Design review of the part built by this model. Coordinates are the model's own, in mm. Face numbers are marked on the shaded views. A direction names the side the tool comes from. Coordinates: 2 decimals unless noted, no trailing zeros. Loops run counter-clockwise (first coordinate to the right, second up) from the corner with the lowest first, then second, coordinate; pieces in that order, holes last. Notation, with made-up numbers: M 44,39.25 L 83,39.25 A25 ccw 83,62.25 Z; hole C 25.25,-19 d3. An arc over 180 degrees is marked long. Answer as a JSON object with one key per item and string values. Group by question number.
1. Draft analysis for pull direction Y (two halves, no side actions). For the marked faces 1, 2 and 3, state which applies: +Y half, -Y half, draft (parallel to the pull), parting line (faces both ways), or undercut.
2. Consider section C-C (z = -3). State the section outline as (x, y) points.
3. Consider section D-D (z = 8.5). State the section outline as (x, y) points, then the cut area to 3 significant figures.
4. Consider section B-B (z = -8). State the section outline as (x, y) points, then the cut area to 3 significant figures.
5. Insertion check: pin 1 (3.5 mm diameter, centred on y = 0, z = -8, fed in from -X); pin 2 (5 mm diameter, centred on y = 20, z = 2, fed in from -X); pin 3 (3 mm diameter, centred on y = -20, z = -3, fed in from -X); pin 4 (10 mm diameter, centred on y = 1, z = -3, fed in from -X). Each pin has a flat end and moves straight along its axis. Give the tip position at first contact, or say it passes through.
6. Machinability: for the marked faces 4 and 5, which of the approach directions +Z, -Z, +X, -X, +Y, -Y give a long, thin tool a straight path to every point of the face, cutting with its end or side? Answer none if there is none.
7. Consider section A-A (x = 0). Count the separate pieces of the cut face and the enclosed holes in it, then the cut area to 3 significant figures.
8. To check wall thickness, follow probe 1 along Z at (x, y) = (-25, 0); probe 2 along Z at (x, y) = (15, -2.5); probe 3 along Z at (x, y) = (-1, 26). State the ranges of each line that lie inside material, in increasing order.
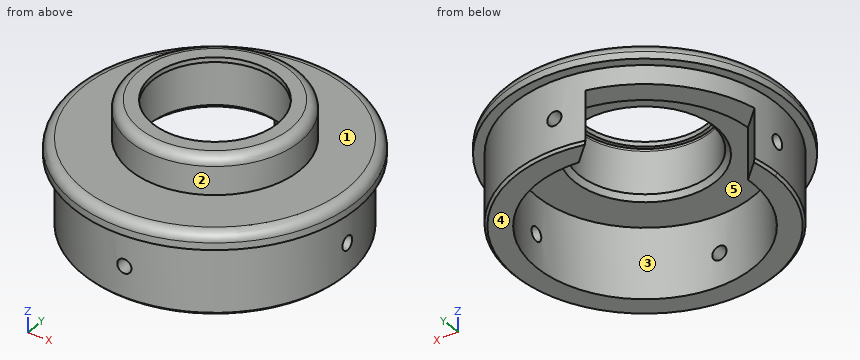
from build123d import *

# Parameters (mm, degrees)
SKETCH_2_R               = 30
SKETCH_2_R_2             = 14
EXTRUDE_1_DEPTH          = 11.5
EXTRUDE_START            = -1.5
SKETCH_3_R               = 14
SKETCH_3_R_2             = 13.25
EXTRUDE_2_DEPTH          = 1.5
SKETCH_4_R               = 33.760613234
SKETCH_4_R_2             = 18
CUT_EXTRUDE_1_DEPTH      = 8
FILLET_1_R               = 2
FILLET_2_R               = 2
SKETCH_6_R               = 28
SKETCH_6_R_2             = 23
EXTRUDE_3_DEPTH          = 15
CUT_EXTRUDE_2_DEPTH      = 46
CUT_EXTRUDE_2_DEPTH_BACK = 46
SKETCH_7_R               = 1.5
CUT_EXTRUDE_3_DEPTH      = 46.000000033
CUT_EXTRUDE_3_DEPTH_BACK = 46.000000033
SKETCH_8_R               = 1.5
CUT_EXTRUDE_4_DEPTH      = 11
SKETCH_15_R              = 14
CUT_EXTRUDE_5_DEPTH      = 0.5
CHAMFER_1_SIZE           = 1
CHAMFER_2_SIZE           = 0.5


with BuildPart() as part:
    # 스케치2 → 보스-돌출1 (new body)
    with BuildSketch(Plane.XY):
        Circle(SKETCH_2_R)
        Circle(SKETCH_2_R_2, mode=Mode.SUBTRACT)
    extrude(amount=EXTRUDE_1_DEPTH)

    # 스케치3 → 보스-돌출2 (add)
    with BuildSketch(Plane.XY.offset(11.5).offset(EXTRUDE_START)):
        Circle(SKETCH_3_R)
        Circle(SKETCH_3_R_2, mode=Mode.SUBTRACT)
    extrude(amount=EXTRUDE_2_DEPTH)

    # 스케치4 → 컷-돌출1 (cut)
    with BuildSketch(Plane.XY.offset(11.5)):
        Circle(SKETCH_4_R)
        Circle(SKETCH_4_R_2, mode=Mode.SUBTRACT)
    extrude(amount=-CUT_EXTRUDE_1_DEPTH, mode=Mode.SUBTRACT)

    # 필렛1
    fillet_1_edges = [part.edges().sort_by_distance(p)[0] for p in [
        (-18, 0, 11.5),
    ]]
    fillet(fillet_1_edges, radius=FILLET_1_R)

    # 필렛2
    fillet_2_edges = [part.edges().sort_by_distance(p)[0] for p in [
        (-30, 0, 3.5),
    ]]
    fillet(fillet_2_edges, radius=FILLET_2_R)

    # 스케치6 → 보스-돌출3 (add)
    with BuildSketch(Plane(origin=(0, 0, 0), x_dir=(-1, 0, 0), z_dir=(0, 0, -1))):
        Circle(SKETCH_6_R)
        Circle(SKETCH_6_R_2, mode=Mode.SUBTRACT)
    extrude(amount=EXTRUDE_3_DEPTH)

    # 스케치7 → 컷-돌출2 (cut, two sides: drawn at the far end of the back side and taken through both)
    with BuildSketch(Plane(origin=(0, 0, 0), x_dir=(1, 0, 0), z_dir=(0, 1, 0)).offset(-CUT_EXTRUDE_2_DEPTH_BACK)):
        with Locations(Location((0, 8, 0), (0, 0, 270))):
            Circle(SKETCH_7_R)
    extrude(amount=CUT_EXTRUDE_2_DEPTH + CUT_EXTRUDE_2_DEPTH_BACK, mode=Mode.SUBTRACT)

    # 스케치8 → 컷-돌출3 (cut, two sides: drawn at the far end of the back side and taken through both)
    with BuildSketch(Plane(origin=(0, 0, 0), x_dir=(0, 0, -1), z_dir=(1, 0, 0)).offset(-CUT_EXTRUDE_3_DEPTH_BACK)):
        with Locations((8, 0)):
            Circle(SKETCH_8_R)
    extrude(amount=CUT_EXTRUDE_3_DEPTH + CUT_EXTRUDE_3_DEPTH_BACK, mode=Mode.SUBTRACT)

    # 스케치13 → 컷-돌출4 (cut)
    with BuildSketch(Plane(origin=(0, 0, -15), x_dir=(-1, 0, 0), z_dir=(0, 0, -1))):
        Polygon((19.798989873, 19.798989873), (30.405591591, 9.192388155), (19.798989873, -1.414213562), (9.192388155, 9.192388155), (-1.414213562, 19.798989873), (9.192388155, 30.405591591), align=None)
    extrude(amount=-CUT_EXTRUDE_4_DEPTH, mode=Mode.SUBTRACT)

    # 스케치15 → 컷-돌출5 (cut)
    with BuildSketch(Plane(origin=(0, 0, 10), x_dir=(-1, 0, 0), z_dir=(0, 0, -1))):
        Circle(SKETCH_15_R)
    extrude(amount=-CUT_EXTRUDE_5_DEPTH, mode=Mode.SUBTRACT)

    # 모따기1
    chamfer_1_edges = [part.edges().sort_by_distance(p)[0] for p in [
        (-14, 0, 0),
    ]]
    chamfer(chamfer_1_edges, length=CHAMFER_1_SIZE)

    # 모따기2
    chamfer_2_edges = [part.edges().sort_by_distance(p)[0] for p in [
        (21.853217724, -17.505338474, -15),
    ]]
    chamfer(chamfer_2_edges, length=CHAMFER_2_SIZE)


solid = part.part
Findings below:
{
 "1": {"face 1": "draft", "face 2": "parting line", "face 3": "undercut"},
 "2": {"outline": "C 0,0 d56; hole C 0,0 d46"},
 "3": {"outline": "C 0,0 d36; hole C 0,0 d28", "area": "402 mm^2"},
 "4": {"outline": "M -27.96,-1.5 A28 ccw -1.5,-27.96 L -1.5,-22.95 A23 cw -22.95,-1.5 Z; M -27.96,1.5 L -22.95,1.5 A23 cw -22.94,1.72 L -27.32,6.11 A28 ccw Z; M -6.11,27.32 L -1.72,22.94 A23 cw -1.5,22.95 L -1.5,27.96 A28 ccw Z; M 1.5,-27.96 A28 ccw 27.96,-1.5 L 22.95,-1.5 A23 cw 1.5,-22.95 Z; M 1.5,22.95 A23 cw 22.95,1.5 L 27.96,1.5 A28 ccw 1.5,27.96 Z", "area": "581 mm^2"},
 "5": {"pin 1": "stops at x = -28", "pin 2": "stops at x = -24.34", "pin 3": "stops at x = -21.02", "pin 4": "stops at x = -30"},
 "6": {"face 4": "-Z, +X, -X, +Y, -Y", "face 5": "-Z"},
 "7": {"separate pieces": "4", "enclosed holes": "0", "area": "293 mm^2"},
 "8": {"probe 1": "z = -15 to -9.5, -6.5 to 3.5", "probe 2": "z = 0 to 11.5", "probe 3": "z = -15 to -9.12, -6.88 to 3.5"}
}
